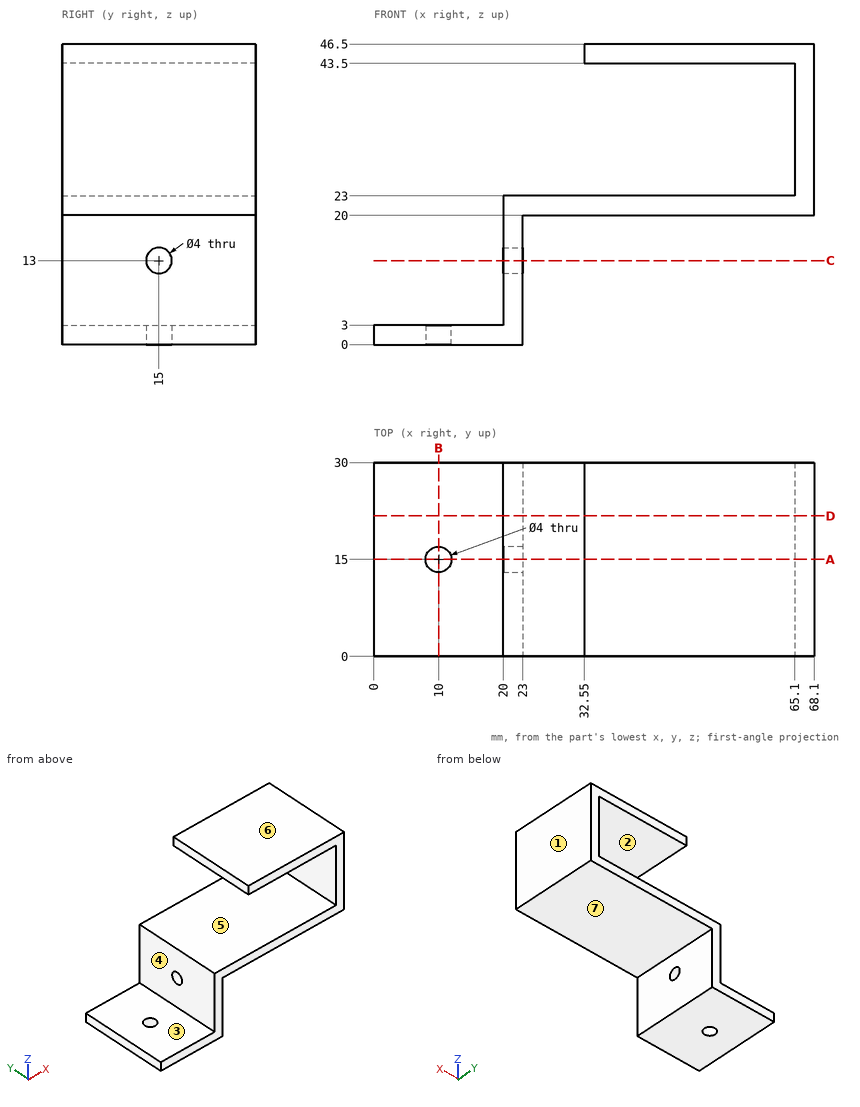
Job drawing, mm, ordinate dimensions from the low corner. One solid piece. A direction names the side the tool comes from. Round coordinates to 2 decimals unless told otherwise and drop trailing zeros. Write each loop counter-clockwise with the first axis right and the second up, starting at its lowest first coordinate (ties: lowest second). Pieces come first, ordered by that corner, then holes. Notation, with made-up numbers: M -17.5,-0.75 L 3.5,-0.75 A16 cw 3.5,17.25 Z; hole C 86.25,19.25 d3. An arc over 180 degrees is marked long. Return JSON: item names as keys, results as strings. Group by question number.
(1) Pin check, flat tips, straight feed: pin 1 Ø3.5 at (y, z) = (15.5, 44.5) entering from -X; pin 2 Ø10 at (x, y) = (48.5, 13) entering from -Z; pin 3 Ø6 at (y, z) = (21.5, 36) entering from -X. Stop position of each tip, or through.
(2) Saw through at C-C on z = 13. Write the cut outline in (x, y), then the cut area to 3 significant figures.
(3) Which spindle directions (+Z, -Z, +X, -X, +Y, -Y) get a long thin tool onto all of the face, cutting with end or side? Do the marked faces 4, 5, 6 and 7. Say none if no direction does.
(4) Drill centre lines: probe 1 along Z at (x, y) = (50, 1.75); probe 2 along X at (y, z) = (15, 2.45); probe 3 along Z at (x, y) = (21.35, 15). Where is each one in solid material? Low to high.
(5) Saw through at B-B on x = 10. Write the cut outline in (y, z), then the cut area to 3 significant figures.
(6) Two-plate mould, pull along Z, no slides. Class the marked faces 1, 2 and 3: +Z half, -Z half, draft (parallel to the pull), parting line (faces both ways), or undercut.
(7) Saw through at A-A on y = 15. Write the cut outline in (x, z), then the cut area to 3 significant figures.
(8) Saw through at D-D on y = 21.75. Write the cut outline in (x, z).
Returned:
{
 "1": {"pin 1": "x = 32.55", "pin 2": "z = 20", "pin 3": "x = 65.1"},
 "2": {"outline": "M 20,0 L 23,0 L 23,13 L 20,13 Z; M 20,17 L 23,17 L 23,30 L 20,30 Z", "area": "78.0 mm²"},
 "3": {"face 4": "+Z, -X, +Y, -Y", "face 5": "-X, +Y, -Y", "face 6": "+Z, +X, -X, +Y, -Y", "face 7": "-Z, +X, +Y, -Y"},
 "4": {"probe 1": "20 to 23, 43.5 to 46.5", "probe 2": "0 to 8, 12 to 23", "probe 3": "0 to 11, 15 to 23"},
 "5": {"outline": "M 0,0 L 13,0 L 13,3 L 0,3 Z; M 17,0 L 30,0 L 30,3 L 17,3 Z", "area": "78.0 mm²"},
 "6": {"face 1": "draft", "face 2": "undercut", "face 3": "+Z half"},
 "7": {"outline": "M 0,0 L 8,0 L 8,3 L 0,3 Z; M 12,0 L 23,0 L 23,11 L 20,11 L 20,3 L 12,3 Z; M 20,15 L 23,15 L 23,20 L 68.1,20 L 68.1,46.5 L 32.55,46.5 L 32.55,43.5 L 65.1,43.5 L 65.1,23 L 20,23 Z", "area": "408 mm²"},
 "8": {"outline": "M 0,0 L 23,0 L 23,20 L 68.1,20 L 68.1,46.5 L 32.55,46.5 L 32.55,43.5 L 65.1,43.5 L 65.1,23 L 20,23 L 20,3 L 0,3 Z"}
}
